Answer from the drawing. Dimensions are ordinates in mm from the lowest x, y and z of the part. A direction names the side the tool comes from. Coordinates: 2 decimals unless noted, no trailing zeros. Write each loop counter-clockwise with the first axis right and the second up, starting at its lowest first coordinate (ties: lowest second). Pieces come first, ordered by that corner, then holes. Notation, with made-up numbers: (-1, -12.75) -> (34, -12.75) arc R27 cw to (34, 24.25) -> close; hole circle Ø4 at (31.25, 47.25). An arc over 180 degrees is marked (long way). One line per item, written item: value. Start each with the question number.
1. Find section C-C, the plane x = 2.5. Write down the section's boundary in (y, z), and give its area (3 significant figures).
2. For the marked faces 1, 2, 3, 4 and 5, determine the directions among +Z, -Z, +X, -X, +Y, -Y from which every point of the face is accessible in a straight line to the end or side of a thin tool.
3. Given P1, Ø1.5, axis at y = 8.5, z = 17, coming from the -X side (1 decimal); P2, Ø0.5, axis at x = 13, y = 3.5, coming from the -Z side; P3, Ø5, axis at x = 2.5, y = 8, coming from the -Z side, each flat-ended and moving along its own axis, determine where each tip first touches the part or whether it passes through.
4. Find section B-B, the plane y = 7.75. Write down the section's boundary in (x, z), and give its area (3 significant figures).
5. Find section A-A, the plane z = 12. Write down the section's boundary in (x, y).
6. Consider line 1 along X through (y, z) = (7.35, 12); line 2 along Z through (x, y) = (13, 5.5); line 3 along Z through (x, y) = (13.5, 8.5). Determine where each line is inside the solid, lowest interval first.
7. Find section D-D, the plane y = 9.25. Write down the section's boundary in (x, z).
8. For a pull along X with two mould halves and no side action, classify the marked faces 6, 7 and 8 as pulls with the +X half, pulls with the -X half, needs draft (parallel to the pull), parting line crosses it, or undercut.
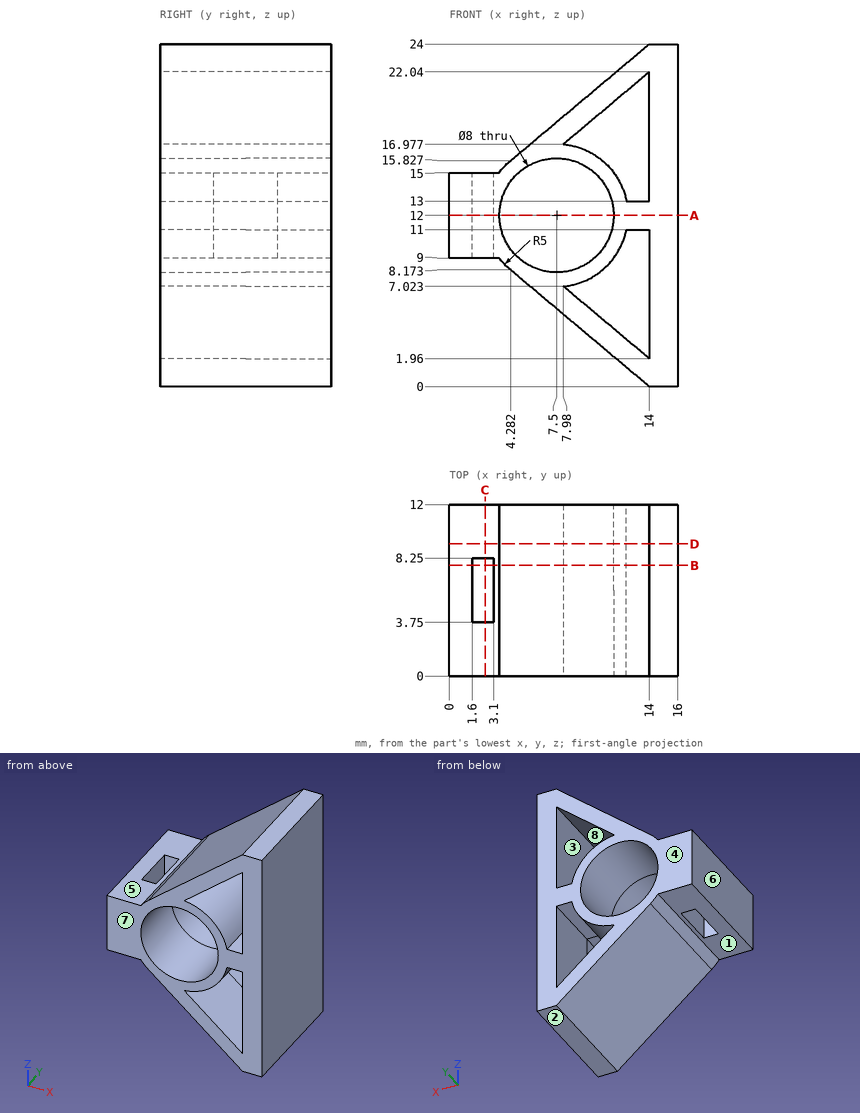
Answer block:
1. outline: (0, 9) -> (3.75, 9) -> (3.75, 15) -> (0, 15) -> close; (8.25, 9) -> (12, 9) -> (12, 15) -> (8.25, 15) -> close
1. area: 45.0 mm2
2. face 1: -Z, -X, +Y, -Y
2. face 2: -Z, +X, -X, +Y, -Y
2. face 3: +Y, -Y
2. face 4: +Z, -Z, +X, -X, +Y
2. face 5: +Z, -X, +Y, -Y
3. P1: stops at x = 4.8
3. P2: stops at z = 0.63
3. P3: stops at z = 7.57
4. outline: (0, 9) -> (1.6, 9) -> (1.6, 15) -> (0, 15) -> close; (3.1, 9) -> (3.5, 9) arc R5 ccw to (4.28, 8.17) -> (14, 0) -> (16, 0) -> (16, 24) -> (14, 24) -> (4.28, 15.83) arc R5 ccw to (3.5, 15) -> (3.1, 15) -> close; hole circle Ø8 at (7.5, 12); hole (7.98, 7.02) -> (14, 1.96) -> (14, 11) -> (12.4, 11) arc R5 cw to start; hole (7.98, 16.98) arc R5 cw to (12.4, 13) -> (14, 13) -> (14, 22.04) -> close
4. area: 116 mm2
5. outline: (0, 0) -> (3.5, 0) -> (3.5, 12) -> (0, 12) -> close; (11.5, 0) -> (16, 0) -> (16, 12) -> (11.5, 12) -> close; hole (1.6, 3.75) -> (3.1, 3.75) -> (3.1, 8.25) -> (1.6, 8.25) -> close
6. line 1: x = 0 to 1.6, 3.1 to 3.5, 11.5 to 16
6. line 2: z = 0.84 to 2.8, 11 to 13, 21.2 to 23.16
6. line 3: z = 0.42 to 2.38, 11 to 13, 21.62 to 23.58
7. outline: (0, 9) -> (3.5, 9) arc R5 ccw to (4.28, 8.17) -> (14, 0) -> (16, 0) -> (16, 24) -> (14, 24) -> (4.28, 15.83) arc R5 ccw to (3.5, 15) -> (0, 15) -> close; hole circle Ø8 at (7.5, 12); hole (7.98, 7.02) -> (14, 1.96) -> (14, 11) -> (12.4, 11) arc R5 cw to start; hole (7.98, 16.98) arc R5 cw to (12.4, 13) -> (14, 13) -> (14, 22.04) -> close
8. face 6: pulls with the -X half
8. face 7: needs draft
8. face 8: undercut
